```python
from build123d import *

# Parameters (mm, degrees)
F1_DEPTH = 76.2
F2_DEPTH = 76.2
F3_DEPTH = 57.15
F5_DEPTH = 25.4
F7_DEPTH = 76.2


with BuildPart() as f1:
    # F0 (on Right) → F1 (new body)
    with BuildSketch(Plane.YZ):
        with BuildLine():
            Line((27.286521, -8.945027), (42.432691, -8.945027))
            ThreePointArc((42.432691, -8.945027), (27.150596, 5.547898), (6.186261, 3.527018))
            ThreePointArc((6.186261, 3.527018), (-0.279827, -1.802061), (-4.66017, -8.945027))
            Line((-4.66017, -8.945027), (10.486, -8.945027))
            ThreePointArc((10.486, -8.945027), (18.886261, -5.770027), (27.286521, -8.945027))
        make_face()
        with BuildLine():
            ThreePointArc((-4.66017, -8.945027), (14.034422, -43.402329), (44.286261, -18.470027))
            ThreePointArc((44.286261, -18.470027), (43.818562, -13.618189), (42.432691, -8.945027))
            Line((42.432691, -8.945027), (27.286521, -8.945027))
            ThreePointArc((27.286521, -8.945027), (30.461521, -13.244767), (31.586261, -18.470027))
            ThreePointArc((31.586261, -18.470027), (13.661, -30.045288), (10.486, -8.945027))
            Line((10.486, -8.945027), (-4.66017, -8.945027))
        make_face()
    extrude(amount=-F1_DEPTH)

    # F0 (on Right) → F2 (join)
    with BuildSketch(Plane.YZ):
        with BuildLine():
            ThreePointArc((42.432691, -8.945027), (43.818562, -13.618189), (44.286261, -18.470027))
            Line((44.286261, -18.470027), (44.286261, 32.329973))
            Line((44.286261, 32.329973), (31.586261, 32.329973))
            Line((31.586261, 32.329973), (31.586261, 19.629973))
            Line((31.586261, 19.629973), (6.186261, 19.629973))
            Line((6.186261, 19.629973), (6.186261, 3.527018))
            ThreePointArc((6.186261, 3.527018), (27.150596, 5.547898), (42.432691, -8.945027))
        make_face()
    extrude(amount=-F2_DEPTH)

    # F0 (on Right) → F3 (cut)
    with BuildSketch(Plane.YZ):
        with BuildLine():
            ThreePointArc((42.432691, -8.945027), (43.818562, -13.618189), (44.286261, -18.470027))
            Line((44.286261, -18.470027), (44.286261, 32.329973))
            Line((44.286261, 32.329973), (31.586261, 32.329973))
            Line((31.586261, 32.329973), (31.586261, 19.629973))
            Line((31.586261, 19.629973), (6.186261, 19.629973))
            Line((6.186261, 19.629973), (6.186261, 3.527018))
            ThreePointArc((6.186261, 3.527018), (27.150596, 5.547898), (42.432691, -8.945027))
        make_face()
    extrude(amount=-F3_DEPTH, mode=Mode.SUBTRACT)

    # F4 (on face) → F5 (cut)
    with BuildSketch(Plane.XZ.offset(-31.586261)):
        Polygon((-76.2, 32.329973), (-66.675, 19.629973), (-57.15, 19.629973), (-57.15, 32.329973), align=None)
    extrude(amount=-F5_DEPTH, mode=Mode.SUBTRACT)

    # F6 (on face) → F7 (cut)
    with BuildSketch(Plane.XZ.offset(-6.186261)):
        Polygon((-57.15, 19.629973), (-66.675, 19.629973), (-57.15, 3.527018), align=None)
    extrude(amount=-F7_DEPTH, mode=Mode.SUBTRACT)


solid = f1.part
```
Design review of the part built by this model. Coordinates are the model's own, in mm. A direction names the side the tool comes from. Round coordinates to 2 decimals unless told otherwise and drop trailing zeros. Order: outer loops, then holes, each group sorted by start corner. A loop starts at its lowest first (then second) coordinate and runs counter-clockwise, first axis right, second up. Notation, with made-up numbers: (39, 43.25) - (61, 43.25) arc R31 ccw to (61, 67.25) - close; hole circle Ø9 at (73, 55.25). An arc over 180 degrees is marked (long way). One line per question, with ' | ' between items.
Item 1: Take a section at A-A, the plane x = -41. Write out the cut boundary in (y, z), then the cut area to 3 significant figures.
Checks:
outline: (-4.66, -8.95) arc R25.4 ccw (long way) to (44.29, -18.47) arc R25.4 ccw to (42.43, -8.95) arc R25.4 ccw to (6.19, 3.53) arc R25.4 ccw to start; hole (27.29, -8.95) arc R12.7 ccw (long way) to (31.59, -18.47) arc R12.7 ccw to start | area: 1,520 mm²
Item 2: For P1, Ø15, axis at y = 18.89, z = -18.47, coming from the +X side; P2, Ø8, axis at x = -15.5, z = -24, coming from the -Y side; P3, Ø13, axis at x = -69.5, z = 15.5, coming from the -Y side; P4, Ø3, axis at x = -72, y = 16, coming from the +Z side, all flat-tipped, find the tip position at first contact; note any pin that passes through.
Checks:
P1: through | P2: y = -6.47 | P3: y = 6.19 | P4: z = 19.63
Item 3: Take a section at D-D, the plane z = -2.5. Write out the cut boundary in (x, y), then the cut area to 3 significant figures.
Checks:
outline: (-76.2, -0.87) - (0, -0.87) - (0, 38.64) - (-57.15, 38.64) - (-57.15, 44.29) - (-76.2, 44.29) - close | area: 3,120 mm²
Item 4: Draft analysis for pull direction X (two halves, no side actions). For faces 1 (the face through (0, 7, -24)), 2 (the face through (-57.15, 19, 5)), 3 (the face through (-69, 6.186, 12)), state which applies: +X half, -X half, draft (parallel to the pull), parting line (faces both ways), or undercut.
Checks:
face 1: +X half | face 2: undercut | face 3: draft
Item 5: Take a section at B-B, the plane z = -19.5. Write out the cut boundary in (x, y).
Checks:
outline: (-76.2, -6.49) - (0, -6.49) - (0, 6.23) - (-76.2, 6.23) - close; (-76.2, 31.54) - (0, 31.54) - (0, 44.27) - (-76.2, 44.27) - close
Item 6: Take a section at C-C, the plane y = 23. Write out the cut boundary in (x, z) (3 decimals), then the cut area to 3 significant figures.
Checks:
outline: (-76.2, -43.535) - (0, -43.535) - (0, -30.485) - (-76.2, -30.485) - close; (-76.2, -6.455) - (0, -6.455) - (0, 6.595) - (-57.15, 6.595) - (-57.15, 3.527) - (-66.675, 19.63) - (-76.2, 19.63) - close | area: 2,160 mm²
Item 7: Machinability: for faces 4 (the face through (-57.15, 41, -2)), 5 (the face through (-71.504, 37.847, 26.069)), 6 (the face through (-72, 19, 19.63)), which of the approach directions +Z, -Z, +X, -X, +Y, -Y give a long, thin tool a straight path to every point of the face, cutting with its end or side? Answer none if there is none.
Checks:
face 4: +Z, +X, +Y | face 5: +Z, +X, +Y, -Y | face 6: +Z, +X, -X, -Y
Item 8: Wall thickness on line 1 (Z direction, x = -20.5, y = 19.5); line 2 (Z direction, x = -51.5, y = 15); line 3 (Y direction, x = -44, z = -9): over which ranges is each line inside the solid? List them lowest first. Write a range as [from, to].
Checks:
line 1: [-43.86, -31.16], [-5.78, 6.92] | line 2: [-43.57, -30.56], [-6.38, 6.63] | line 3: [-4.68, 10.42], [27.35, 42.45]
